```python
from build123d import *


with BuildPart() as part:
    # Esquisse1 → Révolution1 (revolve)
    with BuildSketch(Plane.XY, mode=Mode.PRIVATE) as r_volution1_sk:
        with BuildLine():
            Line((-2, 4), (2, 4))
            Line((2, 4), (2, 5.2))
            Line((2, 5.2), (0.894427191, 5.2))
            ThreePointArc((0.894427191, 5.2), (1.2, 6), (0.894427191, 6.8))
            Line((0.894427191, 6.8), (2, 6.8))
            Line((2, 6.8), (2, 8))
            Line((2, 8), (-2, 8))
            Line((-2, 8), (-2, 6.8))
            Line((-2, 6.8), (-0.894427191, 6.8))
            ThreePointArc((-0.894427191, 6.8), (-1.2, 6), (-0.894427191, 5.2))
            Line((-0.894427191, 5.2), (-2, 5.2))
            Line((-2, 5.2), (-2, 4))
        make_face()
    revolve(r_volution1_sk.sketch.rotate(Axis((-2, 0, 0), (1, 0, 0)), 90), axis=Axis((-2, 0, 0), (1, 0, 0)))


solid = part.part
```
Source: CAD feature listing. Evaluate the final solid. Frame: model axes, mm. Coordinates: 2 decimals unless noted, no trailing zeros. Write each loop counter-clockwise with the first axis right and the second up, starting at its lowest first coordinate (ties: lowest second). Pieces come first, ordered by that corner, then holes. Notation, with made-up numbers: (-32, 7.25) - (-4, 7.25) arc R4 cw to (-4, 13.25) - close; hole circle Ø9 at (32.25, 10). An arc over 180 degrees is marked (long way). Answer as a JSON object with one key per item and string values.
Q1. First-contact query: pin 1 Ø1.5 at (x, y) = (0.5, -3.5) entering from +Z; pin 2 Ø1.5 at (x, z) = (-1, -3.5) entering from +Y; pin 3 Ø2 at (x, y) = (1, 4) entering from +Z. Flat tips, straight axial feed; report the tip coordinate or a pass-through.
Ans:
{"pin 1": "stops at z = 7.51", "pin 2": "stops at y = 7.51", "pin 3": "stops at z = 7.42"}
Q2. Draft query along Y for faces 1 (the cylindrical face through (-0.03, 7.81, -1.73)), 2 (the flat face through (-2, 3, 3)), 3 (the cylindrical face through (0.028, 3.905, -0.867)). Return one class per face: released by +Y, released by -Y, zero draft, split by the parting line, or undercut.
Ans:
{"face 1": "split by the parting line", "face 2": "zero draft", "face 3": "undercut"}
Q3. Section query C-C, the plane x = 0.3. Output: boundary loops of the cut face in (y, z).
Ans:
{"outline": "circle Ø16 at (0, 0); hole circle Ø8 at (0, 0)"}
Q4. Section query A-A, the plane y = 0. Output: boundary loops of the cut face in (x, z), plus the area to 3 significant figures.
Ans:
{"outline": "(-2, -8) - (2, -8) - (2, -6.8) - (0.89, -6.8) arc R1.2 ccw to (0.89, -5.2) - (2, -5.2) - (2, -4) - (-2, -4) - (-2, -5.2) - (-0.89, -5.2) arc R1.2 ccw to (-0.89, -6.8) - (-2, -6.8) - close; (-2, 4) - (2, 4) - (2, 5.2) - (0.89, 5.2) arc R1.2 ccw to (0.89, 6.8) - (2, 6.8) - (2, 8) - (-2, 8) - (-2, 6.8) - (-0.89, 6.8) arc R1.2 ccw to (-0.89, 5.2) - (-2, 5.2) - close", "area": "26.3 mm2"}
Q5. Section query D-D, the plane z = -7. Output: boundary loops of the cut face in (x, y).
Ans:
{"outline": "(-2, -3.87) - (2, -3.87) - (2, 3.87) - (-2, 3.87) - close"}
Q6. Material intervals for line 1 (Y direction, x = -1.35, z = 0); line 2 (Y direction, x = 1.05, z = 0); line 3 (Z direction, x = -1.35, y = 3), sorted ascending. Write a range as [from, to].
Ans:
{"line 1": "y = [-8, -6.8], [-5.2, -4], [4, 5.2], [6.8, 8]", "line 2": "y = [-8, -6.8], [-6.58, -5.42], [-5.2, -4], [4, 5.2], [5.42, 6.58], [6.8, 8]", "line 3": "z = [-7.42, -6.1], [-4.25, -2.65], [2.65, 4.25], [6.1, 7.42]"}
